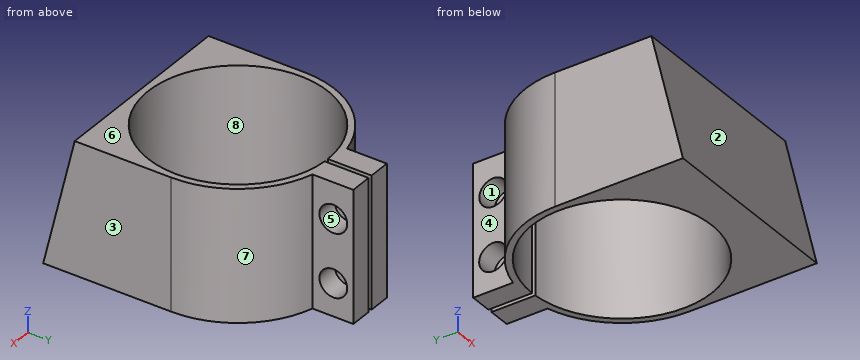
Solid Edge part; units mm, degrees
sketch "Sketch1" plane through (0, 0, 0) normal (0, 0, 1) x (1, 0, 0)
  line L0 (6.0091, 30.5) -> (6.0091, 21.1635)
  line L1 (22.0001, 0) -> (22.0001, -21.9937)
  line L2 (-0.5256, -21.9937) -> (22.0001, -21.9937)
  line L3 (-0.5256, -21.9937) -> (-21.9999, -21.9937)
  line L4 (-21.9999, 0) -> (-21.9999, -21.9937)
  arc A0 (-21.9999, 0) -> (-4.9909, 21.4264) centre (0.0001, 0) cw
  line L5 (-4.9909, 30.5) -> (-4.9909, 21.4264)
  line L6 (0.0091, 30.5) -> (-4.9909, 30.5)
  line L7 (0.0091, 20.5) -> (0.0091, 30.5)
  line L8 (1.0091, 20.5) -> (1.0091, 20.4752)
  line L9 (1.0091, 20.5) -> (1.0091, 30.5)
  line L10 (1.0091, 30.5) -> (6.0091, 30.5)
  arc A1 (6.0091, 21.1635) -> (22.0001, 0) centre (0.0001, 0) cw
  arc A2 (1.0091, 20.4752) -> (0.0091, 20.5) centre (0.0001, 0) cw
extrude "Protrusion1" add sketch "Sketch1" along normal blind 30
hole "Hole_1" at (-4.9909, 25.9632, 7.4167) direction (1, 0, 0) diameter 6.35 end up to next
hole "Hole1" at (-4.9909, 25.9359, 21.8715) direction (1, 0, 0) diameter 6.35 end up to next
hole "Hole_3" at (1.0091, 25.9256, 7.4167) direction (1, 0, 0) diameter 6.35 end up to next
hole "Hole2" at (1.0091, 25.9256, 21.8167) direction (1, 0, 0) diameter 6.35 end up to next
sketch "Sketch2" plane through (22.0001, -10.9968, 15) normal (1, 0, 0) x (0, 1, 0)
  line L0 (-10.9968, 15) -> (-10.9968, -15)
  line L1 (-10.9968, -15) -> (-18.1991, -15)
  line L2 (-10.9968, 15) -> (-18.1991, -15)
extrude "ExtrudedProtrusion_2" add sketch "Sketch2" against normal blind 44
Verification items for the finished model (mm, model axes). Face numbers are marked on the shaded views. A direction names the side the tool comes from. Give positions to 0.01 mm unless a question says otherwise; leave off trailing zeros. Loops run counter-clockwise (first coordinate to the right, second up) from the corner with the lowest first, then second, coordinate; pieces in that order, holes last.
1. Tool access check on the marked faces 1, 2, 3, 4 and 5. Record the directions out of +Z, -Z, +X, -X, +Y, -Y that give a thin tool (end or side, any length) a straight path to the whole face; none if there is none.
Derived:
face 1: -X
face 2: +Z, +X, -X, -Y
face 3: +Z, -Z, +X, +Y, -Y
face 4: +Z, -Z, -X, +Y
face 5: +X
2. Cross-section at B-B on y = -12.5. Record the cut outline in (x, z).
Derived:
outline: (-22, 0) - (-16.25, 0) - (-16.25, 30) - (-22, 30) - close; (16.25, 0) - (22, 0) - (22, 30) - (16.25, 30) - close
3. Go/stop test with flat-tipped pins: P1, Ø2, axis at y = 24.5, z = 5, coming from the +X side; P2, Ø3, axis at y = 28, z = 15.5, coming from the -X side; P3, Ø8, axis at x = 6.5, z = 13, coming from the -Y side. Record where each tip stops, or that it passes through.
Derived:
P1: stops at x = 6.01
P2: stops at x = -4.99
P3: stops at y = -27.04
4. Cross-section at A-A on z = 6.5. Count the separate pieces of the cut face and the enclosed holes in it, and give its area (3 significant figures).
Derived:
separate pieces: 3
enclosed holes: 0
area: 681 mm2
5. Release check for a two-part mould opening along Y. For the marked faces 6, 7 and 8 record: +Y half, -Y half, draft (parallel to the pull), parting line (faces both ways), or undercut.
Derived:
face 6: draft
face 7: +Y half
face 8: undercut
6. Material ranges on probe 1 along X at (y, z) = (22.5, 20); probe 2 along Y at (x, z) = (-2, 23.5); probe 3 along Y at (x, z) = (4, 24.5), recorded low to high.
Derived:
probe 1: x = -4.99 to 0.01, 1.01 to 6.01
probe 2: y = -23.55 to -20.4, 20.4 to 23.21, 28.66 to 30.5
probe 3: y = -23.31 to -20.11, 20.11 to 24.23, 27.62 to 30.5
